```python
from build123d import *

# Parameters (mm, degrees)
BOSS_EXTRUDE1_DEPTH     = 3.175
CUT_EXTRUDE2_DEPTH      = 153.835933275
CUT_EXTRUDE2_DEPTH_BACK = 153.835933275
SKETCH3_R               = 1.25
CUT_EXTRUDE6_DEPTH      = 153.835933275
CUT_EXTRUDE6_DEPTH_BACK = 153.835933275
SKETCH12_R              = 2.25
CUT_EXTRUDE7_DEPTH      = 153.835933275
CUT_EXTRUDE7_DEPTH_BACK = 153.835933275
FILLET4_R               = 4
BOSS_EXTRUDE2_START     = -6.35
SKETCH16_R              = 2.25
BOSS_EXTRUDE2_DEPTH     = 6.35
CUT_EXTRUDE8_DEPTH      = 153.835933275
CUT_EXTRUDE8_DEPTH_BACK = 153.835933275
SKETCH17_R              = 2.25


with BuildPart() as part:
    # Sketch1 → Boss-Extrude1 (new, symmetric)
    with BuildSketch(Plane.XY):
        with BuildLine():
            Line((92.5, 121.5), (-92.5, 121.5))
            Line((-92.5, 121.5), (-92.5, 91.5))
            Line((-92.5, 91.5), (-42.356397926, -19.188161838))
            ThreePointArc((-42.356397926, -19.188161838), (0, -46.5), (42.356397926, -19.188161838))
            Line((42.356397926, -19.188161838), (92.5, 91.5))
            Line((92.5, 91.5), (92.5, 121.5))
        make_face()
    extrude(amount=BOSS_EXTRUDE1_DEPTH, both=True)

    # Sketch3 → Cut-Extrude2 (cut, two sides: drawn at the far end of the back side and taken through both)
    with BuildSketch(Plane(origin=(0, 0, -3.175), x_dir=(-1, 0, 0), z_dir=(0, 0, -1)).offset(-CUT_EXTRUDE2_DEPTH_BACK)):
        with Locations((17.440159599, -16.121517706)):
            Circle(SKETCH3_R)
        with Locations((22.282044228, -8.220280106)):
            Circle(SKETCH3_R)
        with Locations((9.943168767, -21.568400378)):
            Circle(SKETCH3_R)
        with Locations((0.932420624, -23.731689611)):
            Circle(SKETCH3_R)
        with Locations((-8.220280106, -22.282044228)):
            Circle(SKETCH3_R)
        with Locations((-16.121517706, -17.440159599)):
            Circle(SKETCH3_R)
        with Locations((-21.568400378, -9.943168767)):
            Circle(SKETCH3_R)
        with Locations((-23.731689611, -0.932420624)):
            Circle(SKETCH3_R)
        with Locations((-22.282044228, 8.220280106)):
            Circle(SKETCH3_R)
        with Locations((-17.440159599, 16.121517706)):
            Circle(SKETCH3_R)
        with Locations((-9.943168767, 21.568400378)):
            Circle(SKETCH3_R)
        with Locations((-0.932420624, 23.731689611)):
            Circle(SKETCH3_R)
        with Locations((8.220280106, 22.282044228)):
            Circle(SKETCH3_R)
        with Locations((16.121517706, 17.440159599)):
            Circle(SKETCH3_R)
        with Locations((21.568400378, 9.943168767)):
            Circle(SKETCH3_R)
        with Locations((23.731689611, 0.932420624)):
            Circle(SKETCH3_R)
    extrude(amount=CUT_EXTRUDE2_DEPTH + CUT_EXTRUDE2_DEPTH_BACK, mode=Mode.SUBTRACT)

    # Sketch12 → Cut-Extrude6 (cut, two sides: drawn at the far end of the back side and taken through both)
    with BuildSketch(Plane(origin=(0, 0, -3.175), x_dir=(-1, 0, 0), z_dir=(0, 0, -1)).offset(-CUT_EXTRUDE6_DEPTH_BACK)):
        with Locations((-7, 102)):
            Circle(SKETCH12_R)
        with Locations((7, 102)):
            Circle(SKETCH12_R)
        with Locations((7, 116)):
            Circle(SKETCH12_R)
        with Locations((-87, 116)):
            Circle(SKETCH12_R)
        with Locations((-73, 116)):
            Circle(SKETCH12_R)
        with Locations((-73, 102)):
            Circle(SKETCH12_R)
        with Locations((-87, 102)):
            Circle(SKETCH12_R)
        with Locations(Location((87, 102, 0), (0, 0, 180))):
            Circle(SKETCH12_R)
        with Locations(Location((73, 102, 0), (0, 0, 180))):
            Circle(SKETCH12_R)
        with Locations(Location((73, 116, 0), (0, 0, 180))):
            Circle(SKETCH12_R)
        with Locations(Location((87, 116, 0), (0, 0, 180))):
            Circle(SKETCH12_R)
        with Locations((-7, 116)):
            Circle(SKETCH12_R)
    extrude(amount=CUT_EXTRUDE6_DEPTH + CUT_EXTRUDE6_DEPTH_BACK, mode=Mode.SUBTRACT)

    # Sketch13 → Cut-Extrude7 (cut, two sides: drawn at the far end of the back side and taken through both)
    with BuildSketch(Plane(origin=(0, 0, -3.175), x_dir=(-1, 0, 0), z_dir=(0, 0, -1)).offset(-CUT_EXTRUDE7_DEPTH_BACK)):
        with BuildLine():
            Line((-40.739222198, 22.417978828), (-70.6841661, 88.519149462))
            ThreePointArc((-70.6841661, 88.519149462), (-62.939709446, 94.330423107), (-58.354481954, 102.85821292))
            Line((-58.354481954, 102.85821292), (-21.645518046, 102.85821292))
            ThreePointArc((-21.645518046, 102.85821292), (-17.06210253, 94.332530646), (-9.32089354, 88.521451623))
            Line((-9.32089354, 88.521451623), (-9.32089354, 45.556239349))
            ThreePointArc((-9.32089354, 45.556239349), (-27.574418795, 37.441974148), (-40.739222198, 22.417978828))
        make_face()
        with BuildLine():
            Line((40.739222198, 22.417978828), (70.6841661, 88.519149462))
            ThreePointArc((70.6841661, 88.519149462), (62.939709446, 94.330423107), (58.354481954, 102.85821292))
            Line((58.354481954, 102.85821292), (21.645518046, 102.85821292))
            ThreePointArc((21.645518046, 102.85821292), (17.06210253, 94.332530646), (9.32089354, 88.521451623))
            Line((9.32089354, 88.521451623), (9.32089354, 45.556239349))
            ThreePointArc((9.32089354, 45.556239349), (27.574418795, 37.441974148), (40.739222198, 22.417978828))
        make_face()
    extrude(amount=CUT_EXTRUDE7_DEPTH + CUT_EXTRUDE7_DEPTH_BACK, mode=Mode.SUBTRACT)

    # Fillet4
    fillet4_edges = [part.edges().sort_by_distance(p)[0] for p in [
        (-58.354481954, 102.85821292, 0),
        (-70.6841661, 88.519149462, 0),
        (-40.739222198, 22.417978828, 0),
        (-9.32089354, 45.556239349, 0),
        (-9.32089354, 88.521451623, 0),
        (-21.645518046, 102.85821292, 0),
        (70.6841661, 88.519149462, 0),
        (58.354481954, 102.85821292, 0),
        (21.645518046, 102.85821292, 0),
        (9.32089354, 88.521451623, 0),
        (9.32089354, 45.556239349, 0),
        (40.739222198, 22.417978828, 0),
    ]]
    fillet(fillet4_edges, radius=FILLET4_R)

    # Sketch16 → Boss-Extrude2 (add)
    with BuildSketch(Plane.XY.offset(3.175).offset(BOSS_EXTRUDE2_START)):
        with Locations((-87, 102)):
            Circle(SKETCH16_R)
        with Locations((-87, 116)):
            Circle(SKETCH16_R)
        with Locations((-73, 116)):
            Circle(SKETCH16_R)
        with Locations((-73, 102)):
            Circle(SKETCH16_R)
        with Locations((-7, 116)):
            Circle(SKETCH16_R)
        with Locations((7, 116)):
            Circle(SKETCH16_R)
        with Locations((-7, 102)):
            Circle(SKETCH16_R)
        with Locations((7, 102)):
            Circle(SKETCH16_R)
        with Locations((73, 102)):
            Circle(SKETCH16_R)
        with Locations((87, 102)):
            Circle(SKETCH16_R)
        with Locations((73, 116)):
            Circle(SKETCH16_R)
        with Locations((87, 116)):
            Circle(SKETCH16_R)
    extrude(amount=BOSS_EXTRUDE2_DEPTH)

    # Sketch17 → Cut-Extrude8 (cut, two sides: drawn at the far end of the back side and taken through both)
    with BuildSketch(Plane(origin=(0, 0, -3.175), x_dir=(-1, 0, 0), z_dir=(0, 0, -1)).offset(-CUT_EXTRUDE8_DEPTH_BACK)):
        with Locations((78.869644454, 84)):
            Circle(SKETCH17_R)
        with Locations((0, 84)):
            Circle(SKETCH17_R)
        with Locations(Location((-78.869644454, 84, 0), (0, 0, 180))):
            Circle(SKETCH17_R)
        with Locations((0, 109)):
            Circle(SKETCH17_R)
        with Locations((-78.869644454, 109)):
            Circle(SKETCH17_R)
        with Locations((78.869644454, 109)):
            Circle(SKETCH17_R)
    extrude(amount=CUT_EXTRUDE8_DEPTH + CUT_EXTRUDE8_DEPTH_BACK, mode=Mode.SUBTRACT)


solid = part.part
```
The listing builds one solid part. Answer for the finished solid, in the listing's coordinates (mm). A direction names the side the tool comes from. Coordinates: 2 decimals unless noted, no trailing zeros. Loops run counter-clockwise (first coordinate to the right, second up) from the corner with the lowest first, then second, coordinate; pieces in that order, holes last. Notation, with made-up numbers: (82, 67.5) - (117, 67.5) arc R21 ccw to (117, 74.5) - close; hole circle Ø11 at (-23, 0). An arc over 180 degrees is marked (long way). Use a Markdown table: item, result. Add a question column.
1) For faces 5 (the flat face through (-1, 39, 3.175)), 6 (the cylindrical face through (-69.346, 87.965, -0.044)), determine the directions among +Z, -Z, +X, -X, +Y, -Y from which every point of the face is accessible in a straight line to the end or side of a thin tool.
2) The mould has two halves that part along X. Classify faces 1 (the cylindrical face through (-25.78, 38.7, 0.04)), 2 (the cylindrical face through (-0.746, -46.494, 0.044)), 3 (the cylindrical face through (0.488, 106.804, 0.044)), 4 (the flat face through (-1, 39, -3.175)): released by +X, released by -X, zero draft, split by the parting line, or undercut.
3) The part is cut by section D-D, the plane y = 37. Give the vertices of the cut face in (x, z) (3 decimals), and give its area (3 significant figures).
4) Given pin 1 (1.5 mm diameter, centred on y = -2, z = -2.5, fed in from -X); pin 2 (3 mm diameter, centred on y = 71.5, z = -1, fed in from +X), each flat-ended and moving along its own axis, determine where each tip first touches the part or whether it passes through.
5) The part is cut by section B-B, the plane y = 60. Give the vertices of the cut face in (x, z) (3 decimals).
6) The part is cut by section C-C, the plane z = -1.5. State how many separate pieces and enclosed holes the cut face has, and give its area (3 significant figures).
7) The part is cut by section A-A, the plane y = 109. Give the vertices of the cut face in (x, z) (3 decimals), and give its area (3 significant figures).
8) Find the intervals of material crossed by line 1 (X direction, y = 109, z = -0.25); line 2 (X direction, y = 29, z = 1.25); line 3 (Y direction, x = -21, z = 2.5), in increasing order.
Here are the results:
| question | item | result |
|---|---|---|
| 1 | face 5 | +Z, +X, -X, +Y, -Y |
| 1 | face 6 | +Z, -Z |
| 2 | face 1 | undercut |
| 2 | face 2 | split by the parting line |
| 2 | face 3 | undercut |
| 2 | face 4 | zero draft |
| 3 | outline | (-67.811, -3.175) - (-47.345, -3.175) - (-47.345, 3.175) - (-67.811, 3.175) - close; (-28.165, -3.175) - (28.165, -3.175) - (28.165, 3.175) - (-28.165, 3.175) - close; (47.345, -3.175) - (67.811, -3.175) - (67.811, 3.175) - (47.345, 3.175) - close |
| 3 | area | 618 mm^2 |
| 4 | pin 1 | stops at x = -50.48 |
| 4 | pin 2 | stops at x = 84.12 |
| 5 | outline | (-78.23, -3.175) - (-57.765, -3.175) - (-57.765, 3.175) - (-78.23, 3.175) - close; (-9.321, -3.175) - (9.321, -3.175) - (9.321, 3.175) - (-9.321, 3.175) - close; (57.765, -3.175) - (78.23, -3.175) - (78.23, 3.175) - (57.765, 3.175) - close |
| 6 | separate pieces | 1 |
| 6 | enclosed holes | 24 |
| 6 | area | 15,500 mm^2 |
| 7 | outline | (-92.5, -3.175) - (-81.12, -3.175) - (-81.12, 3.175) - (-92.5, 3.175) - close; (-76.62, -3.175) - (-2.25, -3.175) - (-2.25, 3.175) - (-76.62, 3.175) - close; (2.25, -3.175) - (76.62, -3.175) - (76.62, 3.175) - (2.25, 3.175) - close; (81.12, -3.175) - (92.5, -3.175) - (92.5, 3.175) - (81.12, 3.175) - close |
| 7 | area | 1,090 mm^2 |
| 8 | line 1 | x = -92.5 to -81.12, -76.62 to -2.25, 2.25 to 76.62, 81.12 to 92.5 |
| 8 | line 2 | x = -64.19 to -43.72, -36.35 to 36.35, 43.72 to 64.19 |
| 8 | line 3 | y = -41.49 to 8.83, 11.06 to 41.49, 100.83 to 121.5 |
